from build123d import *

# Parameters (mm, degrees)
SKETCH1_W           = 38.1
SKETCH1_H           = 76.2
BOSS_EXTRUDE1_DEPTH = 25.4
SKETCH2_R           = 1.2
CUT_EXTRUDE1_DEPTH  = 3.175
SKETCH4_W           = 34.925
SKETCH4_H           = 73.025
CUT_EXTRUDE2_DEPTH  = 22.225
CUT_EXTRUDE3_DEPTH  = 1.5875
CUT_EXTRUDE4_DEPTH  = 1.5875
SKETCH7_W           = 34.925
SKETCH7_H           = 9.525
CUT_EXTRUDE5_DEPTH  = 1.5875
CUT_EXTRUDE6_DEPTH  = 1.5875
CHAMFER1_SIZE       = 2.54
CHAMFER1_SIZE2      = 0.680590949
CHAMFER3_SIZE       = 2.54
CHAMFER3_SIZE2      = 0.680590949
CHAMFER4_SIZE       = 2.54
CHAMFER4_SIZE2      = 0.680590949
SKETCH10_W          = 6.35
SKETCH10_H          = 0.79375
SKETCH10_W_2        = 4.7625
SKETCH10_H_2        = 0.823022406
CUT_EXTRUDE7_DEPTH  = 4.7625
CUT_EXTRUDE8_REACH  = 88.661
SKETCH11_W          = 6.35
SKETCH11_H          = 1.5875
SKETCH14_W          = 4.7625
SKETCH14_H          = 1.5875
CUT_EXTRUDE9_DEPTH  = 1.5875


with BuildPart() as part:
    # Sketch1 → Boss-Extrude1 (new body)
    with BuildSketch(Plane(origin=(0, 0, 0), x_dir=(1, 0, 0), z_dir=(0, 1, 0))):
        with Locations((-19.05, -38.1)):
            Rectangle(SKETCH1_W, SKETCH1_H)
    extrude(amount=BOSS_EXTRUDE1_DEPTH)

    # Sketch2 → Cut-Extrude1 (cut)
    with BuildSketch(Plane(origin=(0, 0, 0), x_dir=(1, 0, 0), z_dir=(0, 1, 0))):
        with Locations(Location((-33.3375, -4.7625, 0), (0, 0, 270))):
            Circle(SKETCH2_R)
        with Locations(Location((-4.7625, -4.7625, 0), (0, 0, 270))):
            Circle(SKETCH2_R)
        with Locations(Location((-33.3375, -71.4375, 0), (0, 0, 270))):
            Circle(SKETCH2_R)
        with Locations(Location((-4.7625, -71.4375, 0), (0, 0, 270))):
            Circle(SKETCH2_R)
    extrude(amount=CUT_EXTRUDE1_DEPTH, mode=Mode.SUBTRACT)

    # Sketch4 → Cut-Extrude2 (cut)
    with BuildSketch(Plane(origin=(0, 25.4, 0), x_dir=(1, 0, 0), z_dir=(0, 1, 0))):
        with Locations((-19.05, -38.1)):
            Rectangle(SKETCH4_W, SKETCH4_H)
    extrude(amount=-CUT_EXTRUDE2_DEPTH, mode=Mode.SUBTRACT)

    # Sketch5 → Cut-Extrude3 (cut)
    with BuildSketch(Plane.ZY.offset(38.1)):
        with BuildLine():
            Line((76.2, 15.875), (30.115167454, 15.875))
            ThreePointArc((30.115167454, 15.875), (26.9833, 13.9375), (23.851432546, 15.875))
            Line((23.851432546, 15.875), (0, 15.875))
            Line((0, 15.875), (0, 25.4))
            Line((0, 25.4), (76.2, 25.4))
            Line((76.2, 25.4), (76.2, 15.875))
        make_face()
    extrude(amount=-CUT_EXTRUDE3_DEPTH, mode=Mode.SUBTRACT)

    # Sketch6 → Cut-Extrude4 (cut)
    with BuildSketch(Plane(origin=(0, 0, 0), x_dir=(-1, 0, 0), z_dir=(0, 0, -1))):
        with BuildLine():
            Line((30.0117, 12.8875), (30.0117, 15.875))
            Line((30.0117, 15.875), (36.5125, 15.875))
            Line((36.5125, 15.875), (36.5125, 25.4))
            Line((36.5125, 25.4), (1.5875, 25.4))
            Line((1.5875, 25.4), (1.5875, 15.7025))
            Line((1.5875, 15.7025), (9.4717, 15.7025))
            ThreePointArc((9.4717, 15.7025), (12.6467, 12.5275), (15.8217, 15.7025))
            Line((15.8217, 15.7025), (17.4117, 15.7025))
            Line((17.4117, 15.7025), (17.4117, 12.8875))
            Line((17.4117, 12.8875), (20.2117, 12.8875))
            Line((20.2117, 12.8875), (20.2117, 10.9375))
            Line((20.2117, 10.9375), (27.2117, 10.9375))
            Line((27.2117, 10.9375), (27.2117, 12.8875))
            Line((27.2117, 12.8875), (30.0117, 12.8875))
        make_face()
    extrude(amount=-CUT_EXTRUDE4_DEPTH, mode=Mode.SUBTRACT)

    # Sketch7 → Cut-Extrude5 (cut)
    with BuildSketch(Plane.XY.offset(76.2)):
        with Locations((-19.05, 20.6375)):
            Rectangle(SKETCH7_W, SKETCH7_H)
    extrude(amount=-CUT_EXTRUDE5_DEPTH, mode=Mode.SUBTRACT)

    # Sketch8 → Cut-Extrude6 (cut)
    with BuildSketch(Plane(origin=(0, 0, 0), x_dir=(0, 0, -1), z_dir=(1, 0, 0))):
        Polygon((-76.2, 25.4), (-76.2, 15.875), (-31.0375, 15.875), (-31.0375, 11.73125), (-22.0375, 11.73125), (-22.0375, 15.875), (-17.913122854, 15.875), (-17.913122854, 13.4775), (-15.633122854, 13.4775), (-15.628122854, 11.9775), (-10.038122854, 11.9775), (-10.033122854, 13.4775), (-7.753122854, 13.4775), (-7.753122854, 15.7025), (0, 15.7025), (0, 15.875), (0, 25.4), align=None)
    extrude(amount=-CUT_EXTRUDE6_DEPTH, mode=Mode.SUBTRACT)

    # Chamfer1
    chamfer1_edges = [part.edges().sort_by_distance(p)[0] for p in [
        (-38.1, 13.9375, 26.9833),
    ]]
    chamfer1_side = [part.faces().sort_by_distance(p)[0] for p in [
        (-38.1, 7.88589412, 38.18034211),
    ]]
    chamfer(chamfer1_edges, length=CHAMFER1_SIZE, length2=CHAMFER1_SIZE2, reference=chamfer1_side[0])

    # Chamfer3
    chamfer3_edges = [part.edges().sort_by_distance(p)[0] for p in [
        (-20.2117, 11.9125, 0),
        (-23.7117, 10.9375, 0),
        (-27.2117, 11.9125, 0),
    ]]
    chamfer3_side = [part.faces().sort_by_distance(p)[0] for p in [
        (-18.850549312, 7.148250007, 0),
    ]]
    chamfer(chamfer3_edges, length=CHAMFER3_SIZE, length2=CHAMFER3_SIZE2, reference=chamfer3_side[0])

    # Chamfer4
    chamfer4_edges = [part.edges().sort_by_distance(p)[0] for p in [
        (0, 12.7275, 10.035622854),
        (0, 12.7275, 15.630622854),
        (0, 11.9775, 12.833122854),
    ]]
    chamfer4_side = [part.faces().sort_by_distance(p)[0] for p in [
        (0, 7.556578666, 39.246012672),
    ]]
    chamfer(chamfer4_edges, length=CHAMFER4_SIZE, length2=CHAMFER4_SIZE2, reference=chamfer4_side[0])

    # Sketch10 → Cut-Extrude7 (cut)
    with BuildSketch(Plane(origin=(0, 15.875, 0), x_dir=(1, 0, 0), z_dir=(0, 1, 0))):
        with Locations((-30.1625, -75.009375)):
            Rectangle(SKETCH10_W, SKETCH10_H)
        with Locations((-33.3375, -1.190625)):
            Rectangle(SKETCH10_W_2, SKETCH10_H)
        with Locations((-4.7625, -1.190625)):
            Rectangle(SKETCH10_W_2, SKETCH10_H)
        with Locations((-7.9375, -75.024011203)):
            Rectangle(SKETCH10_W, SKETCH10_H_2)
    extrude(amount=-CUT_EXTRUDE7_DEPTH, mode=Mode.SUBTRACT)

    # Sketch11 → Cut-Extrude8 (cut, up to next)
    with BuildSketch(Plane.XY.offset(76.2), mode=Mode.PRIVATE) as cut_extrude8_sk1:
        with Locations((-30.1625, 11.90625)):
            Rectangle(SKETCH11_W, SKETCH11_H)
    cut_extrude8_tool1 = extrude(cut_extrude8_sk1.sketch, amount=-CUT_EXTRUDE8_REACH, mode=Mode.PRIVATE) & part.part
    # Sketch11 → Cut-Extrude8 (cut, up to next)
    with BuildSketch(Plane.XY.offset(76.2), mode=Mode.PRIVATE) as cut_extrude8_sk2:
        with Locations((-7.9375, 11.90625)):
            Rectangle(SKETCH11_W, SKETCH11_H)
    cut_extrude8_tool2 = extrude(cut_extrude8_sk2.sketch, amount=-CUT_EXTRUDE8_REACH, mode=Mode.PRIVATE) & part.part
    add(cut_extrude8_tool1.solids().sort_by_distance((-30.1625, 11.90625, 76.2))[0], mode=Mode.SUBTRACT)
    add(cut_extrude8_tool2.solids().sort_by_distance((-7.9375, 11.90625, 76.2))[0], mode=Mode.SUBTRACT)

    # Sketch14 → Cut-Extrude9 (cut)
    with BuildSketch(Plane(origin=(0, 0, 0), x_dir=(-1, 0, 0), z_dir=(0, 0, -1))):
        with Locations((33.3375, 11.90625)):
            Rectangle(SKETCH14_W, SKETCH14_H)
        with Locations((4.7625, 11.90625)):
            Rectangle(SKETCH14_W, SKETCH14_H)
    extrude(amount=-CUT_EXTRUDE9_DEPTH, mode=Mode.SUBTRACT)


solid = part.part
The model under review builds one solid part; all positions refer to its coordinate system, in mm. A direction names the side the tool comes from. Coordinates: 2 decimals unless noted, no trailing zeros. Loops run counter-clockwise (first coordinate to the right, second up) from the corner with the lowest first, then second, coordinate; pieces in that order, holes last.
(1) Consider section A-A, the plane x = -8. Give the boundary of the cut face in (y, z) (1 decimal), plus the area to 3 significant figures.
Determined:
outline: (0, 0) - (15.7, 0) - (15.7, 1.6) - (3.2, 1.6) - (3.2, 74.6) - (11.1, 74.6) - (11.1, 76.2) - (0, 76.2) - close; (12.7, 75.4) - (15.9, 75.4) - (15.9, 76.2) - (12.7, 76.2) - close
area: 277 mm2
(2) Consider section B-B, the plane y = 4.5. Give the boundary of the cut face in (x, z).
Determined:
outline: (-38.1, 0) - (0, 0) - (0, 76.2) - (-38.1, 76.2) - close; hole (-36.51, 1.59) - (-1.59, 1.59) - (-1.59, 74.61) - (-36.51, 74.61) - close
(3) Wall thickness on L1, parallel to Z at x = -11, y = 6.5; L2, parallel to X at y = 7, z = 16.5; L3, parallel to Z at x = -32.5, y = 15: over which ranges is each line inside the solid? List them lowest first.
Determined:
L1: z = 0 to 1.59, 74.61 to 76.2
L2: x = -38.1 to -36.51, -1.59 to 0
L3: z = 0 to 0.79, 75.41 to 76.2
(4) Insertion check: P1, Ø1.5, axis at x = -9, z = 28.5, coming from the +Y side (3 decimals); P2, Ø0.5, axis at x = -30, z = 75, coming from the +Y side; P3, Ø1.3, axis at x = -28.5, z = 0.5, coming from the +Y side; P4, Ø1.9, axis at x = -33.34, z = 4.76, coming from the -Y side. Each pin has a flat end and moves straight along its axis. Give the tip position at first contact, or say it passes through.
Determined:
P1: stops at y = 3.175
P2: stops at y = 11.11
P3: stops at y = 12.89
P4: passes through
(5) Consider section C-C, the plane z = 55.5. Give the boundary of the cut face in (x, y) (1 decimal), plus the area to 3 significant figures.
Determined:
outline: (-38.1, 0) - (0, 0) - (0, 15.9) - (-1.6, 15.9) - (-1.6, 3.2) - (-36.5, 3.2) - (-36.5, 15.9) - (-38.1, 15.9) - close
area: 161 mm2
(6) Draft analysis for pull direction X (two halves, no side actions). For faces 6 (the flat face through (-33.338, 13, 75)), 7 (the conical face through (-37.53, 13.53, 27.05)), 8 (the cylindrical face through (-36.972, 13.938, 27.038)), state which applies: +X half, -X half, draft (parallel to the pull), parting line (faces both ways), or undercut.
Determined:
face 6: undercut
face 7: -X half
face 8: draft
(7) Tool access review of faces 1 (the flat face through (-1, 11.731, 27)), 2 (the flat face through (-17, 15.702, 1)), 3 (the flat face through (-7.144, 13, 1)), 4 (the flat face through (-19, 10, 74.613)), 5 (the flat face through (-33, 11.112, 1)): name each direction out of +Z, -Z, +X, -X, +Y, -Y from which nothing blocks a thin tool from reaching the whole face with its end or side.
Determined:
face 1: +X, +Y
face 2: -Z, +X, +Y
face 3: none
face 4: +Y
face 5: -Z
